For this review, take the finished solid that the model builds, in its own axes (mm). A direction names the side the tool comes from. Coordinates: 2 decimals unless noted, no trailing zeros. Write each loop counter-clockwise with the first axis right and the second up, starting at its lowest first coordinate (ties: lowest second). Pieces come first, ordered by that corner, then holes. Notation, with made-up numbers: (-24.5, 63.25) -> (29.5, 63.25) arc R31 cw to (29.5, 92.25) -> close; hole circle Ø11 at (24, 39). An arc over 180 degrees is marked (long way). One line per item, written item: value. Start each with the question number.
1) For probe 1 along Y at (x, z) = (3.25, 0) (3 decimals); probe 2 along Y at (x, z) = (2.25, 2); probe 3 along Y at (x, z) = (2.5, 11), list the stretches that pass through material, from the lowest coordinate up. Write a range as from..to.
2) Add section D-D (y = 130). State the section outline as (x, z) points.
3) Mouldability with a two-part tool opening along Z and no side actions: class faces 3 (the flat face through (3, 91, 25.4)), 4 (the cylindrical face through (3.131, 148.684, -0.413)), 5 (the cylindrical face through (3.131, 158.235, 0.357)) as released by +Z, released by -Z, zero draft, split by the parting line, or undercut.
4) Add section B-B (y = 0). State the section outline as (x, z) points (3 decimals).
5) For pin 1 Ø3 at (x, y) = (4.5, 76) entering from -Z; pin 2 Ø4 at (y, z) = (20.62, 11.91) entering from -X, all flat-tipped, find the tip position at first contact; note any pin that passes through.
6) Add section A-A (z = 0). State the section outline as (x, y) points (3 decimals), and give its area (3 significant figures).
7) Machinability: for faces 1 (the cylindrical face through (3.131, -15.497, -3.441)), 2 (the flat face through (3, 91, -25.4)), which of the approach directions +Z, -Z, +X, -X, +Y, -Y give a long, thin tool a straight path to every point of the face, cutting with its end or side? Answer none if there is none.
8) Add section C-C (x = 5.25). State how many separate pieces and enclosed holes the cut face has, and give its area (3 significant figures).
Autodesk Inventor part; units mm, degrees
ref_plane "YZ Plane" through (0, 0, 0) normal (1, 0, 0) x (0, 1, 0)
ref_plane "XZ Plane" through (0, 0, 0) normal (0, 1, 0) x (-1, 0, 0)
ref_plane "XY Plane" through (0, 0, 0) normal (0, 0, 1) x (1, 0, 0)
sketch "Sketch1" plane through (0, 0, 0) normal (1, 0, 0) x (0, 1, 0)
  circle A0 centre (0, 0) radius 158.2356
  dimension "d0" = 316.4711
extrude "Extrusion1" add sketch "Sketch1" along normal blind 6.35
sketch "Sketch2" plane through (0, 0, 0) normal (-1, 0, 0) x (0, 0, 1)
  circle A0 centre (0, 145.5356) radius 3.175
  point P0 (0, 0)
  dimension "d3" = 6.35
  dimension "d4" = 145.5356
extrude "Extrusion2" cut sketch "Sketch2" against normal through all
sketch "Sketch3" plane through (0, 0, 0) normal (-1, 0, 0) x (0, 0, 1)
  point P0 (0, 0)
  point P1 (23.8125, 0)
  point P2 (11.9063, 20.6222)
  point P3 (-11.9062, 20.6222)
  point P4 (-23.8125, 0)
  point P5 (-11.9063, -20.6222)
  point P6 (11.9062, -20.6222)
  dimension "d7" = 23.8125
  dimension "d10" = 360
hole "Hole1" at (0, 0, 23.8125) at (0, 20.6222, 11.9063) at (0, 20.6222, -11.9062) at (0, 0, -23.8125) at (0, -20.6222, -11.9063) at (0, -20.6222, 11.9062) direction (1, 0, 0) diameter 4.4958 end through all
sketch "Sketch4" plane through (0, 0, 0) normal (-1, 0, 0) x (0, 0, 1)
  circle A0 centre (0, 0) radius 15.875
  dimension "d19" = 31.75
extrude "Extrusion3" cut sketch "Sketch4" against normal through all
sketch "Sketch6" plane through (0, 0, 0) normal (-1, 0, 0) x (0, 0, 1)
  arc A0 (-25.4, 28.3981) -> (25.4, 28.3981) centre (0, 0) ccw
  line L0 (-25.4, 28.3981) -> (-25.4, 156.1837)
  circle A1 centre (0, 0) radius 158.2356
  line L1 (25.4, 28.3981) -> (25.4, 156.1837)
  dimension "d29" = 25.4
  dimension "d30" = 25.4
  dimension "d31" = 76.2
extrude "Extrusion4" cut sketch "Sketch6" against normal through all contours A0 L1 A1 L0 picked at (-31.115, 112.3302)
equation "\"d0\" = camPlateDiam"
equation "\"d1\" = camPlateThickness"
equation "\"d3\" = camPostHoleDiam"
equation "\"d5\" = camPlateThickness"
equation "\"d19\" = centerHoleDiam"
equation "\"camPlateThickness\" = 6.35"
equation "\"camPostHoleDiam\" = 6.35"
equation "\"camPostHeight\" = 25.4"
equation "\"camRadius\" = 0.5 * camDiam"
equation "\"aM6HoleDiam\" = 47.625"
equation "\"am6HoleRadius\" = 0.5 * aM6HoleDiam"
equation "\"centerHoleDiam\" = 31.75"
equation "\"camStroke\" = 152.4"
equation "\"pi\" = 79.7941"
properties part number "camPlateCircular" material "Aluminum 6061"
Numbers:
1. probe 1: -38.1..-15.875, 15.875..142.361, 148.711..158.236
1. probe 2: -38.05..-15.75, 15.75..143.07, 148..158.22
1. probe 3: -36.48..-22.68, -18.57..-11.45, 11.45..18.57, 22.68..157.85
2. outline: (0, -25.4) -> (6.35, -25.4) -> (6.35, 25.4) -> (0, 25.4) -> close
3. face 3: released by +Z
3. face 4: undercut
3. face 5: split by the parting line
4. outline: (0, -38.1) -> (6.35, -38.1) -> (6.35, -26.06) -> (0, -26.06) -> close; (0, -21.565) -> (6.35, -21.565) -> (6.35, -15.875) -> (0, -15.875) -> close; (0, 15.875) -> (6.35, 15.875) -> (6.35, 21.565) -> (0, 21.565) -> close; (0, 26.06) -> (6.35, 26.06) -> (6.35, 38.1) -> (0, 38.1) -> close
5. pin 1: z = -25.4
5. pin 2: through
6. outline: (0, -38.1) -> (6.35, -38.1) -> (6.35, -15.875) -> (0, -15.875) -> close; (0, 15.875) -> (6.35, 15.875) -> (6.35, 142.361) -> (0, 142.361) -> close; (0, 148.711) -> (6.35, 148.711) -> (6.35, 158.236) -> (0, 158.236) -> close
6. area: 1,000 mm²
7. face 1: +X, -X
7. face 2: -Z, +X, -X, +Y
8. separate pieces: 1
8. enclosed holes: 8
8. area: 9,860 mm²
